Can you work these out from the model? Positions are in its coordinate system, mm. A direction names the side the tool comes from. Round coordinates to 2 decimals unless told otherwise and drop trailing zeros. Order: outer loops, then holes, each group sorted by start corner. A loop starts at its lowest first (then second) coordinate and runs counter-clockwise, first axis right, second up. Notation, with made-up numbers: (32.5, 29.5) -> (82.5, 29.5) arc R15 ccw to (82.5, 41.5) -> close; hole circle Ø9 at (54, 41). An arc over 180 degrees is marked (long way). Use a Markdown table: item, result. Add a question column.
Q1. If we section it at C-C on y = -30: List the corners of the cut face in (x, z) for me, plus the area to 3 significant figures.
Q2. If we section it at A-A on x = 0: List the corners of the cut face in (y, z) for me, plus the area to 3 significant figures.
Q3. I'm going to push flat-ended pins straight in: pin 1 Ø6 at (y, z) = (9.5, -27.5) entering from -X; pin 2 Ø4 at (y, z) = (23, 0.5) entering from +X; pin 3 Ø1.5 at (x, y) = (15, 33.5) entering from +Z; pin 4 Ø8 at (x, z) = (0, 0) entering from +Y. Where does each tip first touch, or does it pass through?
Q4. We'd pull the mould along X, two halves only. Please class faces 4 (the face through (42.245, 34.715, 21.973)), 5 (the face through (-11.49, -13.784, -1.509)), 6 (the face through (-5, -67.371, -2)): +X half, -X half, draft (parallel to the pull), parting line (faces both ways), or undercut.
Q5. For faces 1 (the face through (37.809, 35.736, 19.665)), 2 (the face through (4.496, -43.509, 2.338)), 3 (the face through (6.126, -44.559, -7.989)), which set-ups out of +Z, -Z, +X, -X, +Y, -Y let a thin tool reach every point of the face, with its end or its side?
Q6. If we section it at D-D on y = 27: List the corners of the cut face in (x, z) for me, plus the area to 3 significant figures.
Q7. If we section it at B-B on z = 0: List the corners of the cut face in (x, y) for me.
Q8. I need wall thicknesses on line 1 along X through (y, z) = (-51.5, 0); line 2 along X through (y, z) = (34, 0); line 3 along Z through (x, y) = (34, 32). Which ranges of each line are inside material? Lowest first, please. Write a range as [from, to].
```python
from build123d import *

# Parameters (mm, degrees)
VACIADO1_T = -5


with BuildPart() as part:
    # Croquis1 → Revolución1 (revolve)
    with BuildSketch(Plane(origin=(0, 0, 0), x_dir=(0, 0, -1), z_dir=(1, 0, 0)), mode=Mode.PRIVATE) as revoluci_n1_sk:
        Polygon((0, 53.716293677), (0, -67.370540613), (10.067532341, -67.370540613), (10.067532341, -22.376525686), (47.617684505, 15.173626478), (47.617684505, 53.716293677), align=None)
    revolve(revoluci_n1_sk.sketch.rotate(Axis((0, 53.716293677, 0), (0, -1, 0)), 180), axis=Axis((0, 53.716293677, 0), (0, -1, 0)))

    # Vaciado1
    vaciado1_openings = [part.faces().sort_by_distance(p)[0] for p in [
        (0, -67.370540613, 0),
        (0, 53.716293677, 0),
    ]]
    offset(amount=VACIADO1_T, openings=vaciado1_openings, kind=Kind.INTERSECTION)


solid = part.part
```
Answer below:
| question | item | result |
|---|---|---|
| 1 | outline | circle Ø20.14 at (0, 0); hole circle Ø10.14 at (0, 0) |
| 1 | area | 238 mm² |
| 2 | outline | (-67.37, -10.07) -> (-22.38, -10.07) -> (15.17, -47.62) -> (53.72, -47.62) -> (53.72, -42.62) -> (17.24, -42.62) -> (-20.31, -5.07) -> (-67.37, -5.07) -> close; (-67.37, 5.07) -> (-20.31, 5.07) -> (17.24, 42.62) -> (53.72, 42.62) -> (53.72, 47.62) -> (15.17, 47.62) -> (-22.38, 10.07) -> (-67.37, 10.07) -> close |
| 2 | area | 1,370 mm² |
| 3 | pin 1 | x = -36.17 |
| 3 | pin 2 | x = 47.62 |
| 3 | pin 3 | z = 45.44 |
| 3 | pin 4 | through |
| 4 | face 4 | parting line |
| 4 | face 5 | undercut |
| 4 | face 6 | draft |
| 5 | face 1 | +Y |
| 5 | face 2 | +Y, -Y |
| 5 | face 3 | -Y |
| 6 | outline | circle Ø95.24 at (0, 0); hole circle Ø85.24 at (0, 0) |
| 6 | area | 1,420 mm² |
| 7 | outline | (-47.62, 15.17) -> (-10.07, -22.38) -> (-10.07, -67.37) -> (-5.07, -67.37) -> (-5.07, -20.31) -> (-42.62, 17.24) -> (-42.62, 53.72) -> (-47.62, 53.72) -> close; (5.07, -67.37) -> (10.07, -67.37) -> (10.07, -22.38) -> (47.62, 15.17) -> (47.62, 53.72) -> (42.62, 53.72) -> (42.62, 17.24) -> (5.07, -20.31) -> close |
| 8 | line 1 | [-10.07, -5.07], [5.07, 10.07] |
| 8 | line 2 | [-47.62, -42.62], [42.62, 47.62] |
| 8 | line 3 | [-33.34, -25.7], [25.7, 33.34] |
